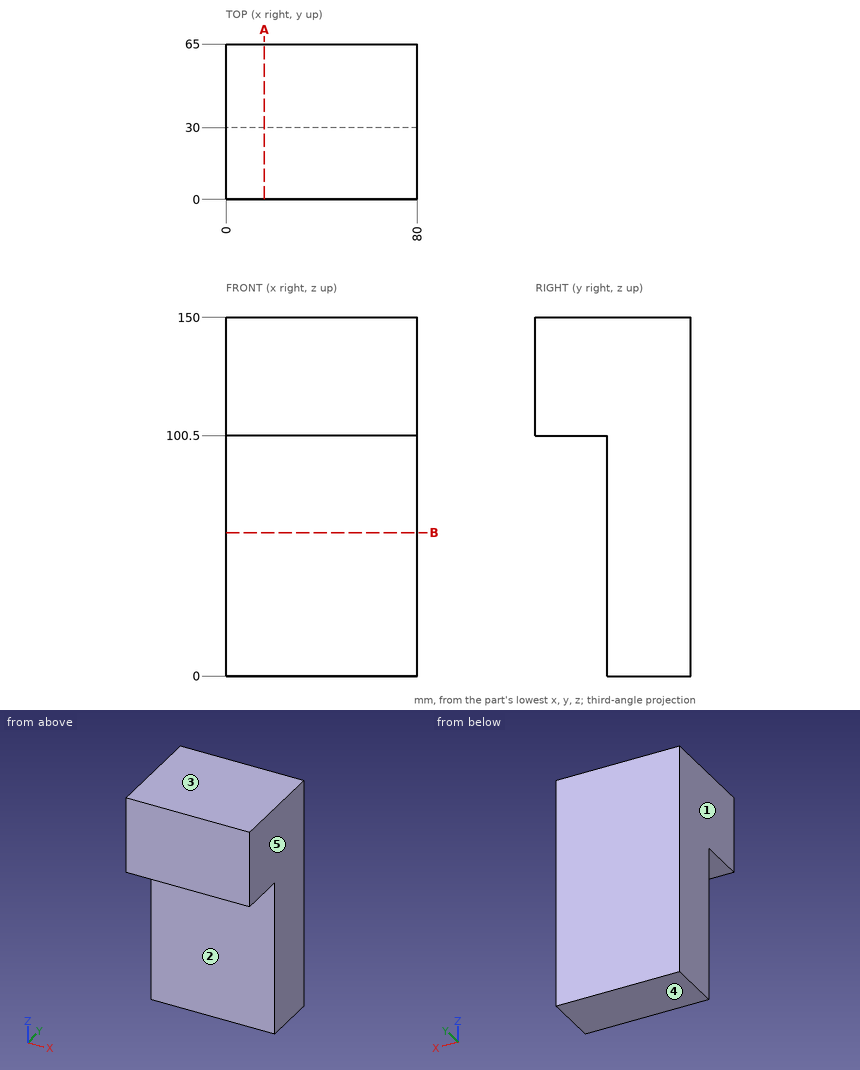
Could you check a few things on this drawing? It's one solid part, dimensions in mm from its lowest x, y, z. A direction names the side the tool comes from. Give positions to 0.01 mm unless a question says otherwise; leave off trailing zeros. Loops run counter-clockwise (first coordinate to the right, second up) from the corner with the lowest first, then second, coordinate; pieces in that order, holes last. Notation, with made-up numbers: M -11,-24.75 L -7,-24.75 A13 cw -7,-2.75 Z; hole C 39,72 d5. An arc over 180 degrees is marked long. Return JSON: item names as keys, results as strings.
Item 1: I'm going to push a flat-ended pin straight in: pin 1 Ø2 at (x, z) = (52.5, 69.5) entering from -Y. Where does the tip first touch, or does it pass through?
A:
{"pin 1": "stops at y = 30"}
Item 2: Please list where these lines run through material, in increasing order: line 1 (Z direction, x = 37, y = 23); line 2 (Y direction, x = 40.5, z = 6.5).
A:
{"line 1": "z = 100.5 to 150", "line 2": "y = 30 to 65"}
Item 3: On a 3-axis mill with a long thin cutter (end or side, diameter ignored), from which of +Z, -Z, +X, -X, +Y, -Y can I reach the whole of each face in a straight line? I mean the marked faces 1 and 2. Say none if no direction works.
A:
{"face 1": "+Z, -Z, -X, +Y, -Y", "face 2": "-Z, +X, -X, -Y"}
Item 4: Imagine slicing it at A-A on x = 16. List the corners of the cut face in (y, z) for me, then the cut area to 4 significant figures.
A:
{"outline": "M 0,100.5 L 30,100.5 L 30,0 L 65,0 L 65,150 L 0,150 Z", "area": "6,735 mm^2"}
Item 5: Thinking about a two-plate mould opening in Z: for the marked faces 3, 4 and 5, which applies, released by +Z, released by -Z, zero draft, split by the parting line, or undercut?
A:
{"face 3": "released by +Z", "face 4": "released by -Z", "face 5": "zero draft"}
Item 6: Imagine slicing it at B-B on z = 60. List the corners of the cut face in (x, y) for me, then the cut area to 3 significant figures.
A:
{"outline": "M 0,30 L 80,30 L 80,65 L 0,65 Z", "area": "2,800 mm^2"}
